from build123d import *

# Parameters (mm, degrees)
F0_R     = 2.3495
F0_R_2   = 3.96875
F0_W     = 15.748
F0_H     = 17.272
F0_W_2   = 48.387
F0_H_2   = 25.781
F0_R_3   = 7.14375
F1_DEPTH = 6.35


with BuildPart() as f1:
    # F0 (on Top) → F1 (new body)
    with BuildSketch(Plane.XY):
        with BuildLine():
            ThreePointArc((61.595, 55.245), (59.735128, 59.735128), (55.245, 61.595))
            Line((55.245, 61.595), (-55.245, 61.595))
            ThreePointArc((-55.245, 61.595), (-59.735128, 59.735128), (-61.595, 55.245))
            Line((-61.595, 55.245), (-61.595, -55.245))
            ThreePointArc((-61.595, -55.245), (-59.735128, -59.735128), (-55.245, -61.595))
            Line((-55.245, -61.595), (55.245, -61.595))
            ThreePointArc((55.245, -61.595), (59.735128, -59.735128), (61.595, -55.245))
            Line((61.595, -55.245), (61.595, 55.245))
        make_face()
        with Locations((-45.212, -41.402)):
            Circle(F0_R, mode=Mode.SUBTRACT)
        with Locations((-29.845, -23.495)):
            Circle(F0_R_2, mode=Mode.SUBTRACT)
        with Locations((10.795, -33.02)):
            Circle(F0_R_2, mode=Mode.SUBTRACT)
        with Locations((45.212, -41.402)):
            Circle(F0_R, mode=Mode.SUBTRACT)
        with Locations((29.845, -23.495)):
            Circle(F0_R_2, mode=Mode.SUBTRACT)
        with Locations((10.795, -13.97)):
            Circle(F0_R_2, mode=Mode.SUBTRACT)
        with Locations((-29.845, 20.32)):
            Rectangle(F0_W, F0_H, mode=Mode.SUBTRACT)
        with Locations((-45.212, 41.402)):
            Circle(F0_R, mode=Mode.SUBTRACT)
        with Locations((10.795, 20.32)):
            Rectangle(F0_W_2, F0_H_2, mode=Mode.SUBTRACT)
        with Locations((0, 50.224401)):
            Circle(F0_R_3, mode=Mode.SUBTRACT)
        with Locations((45.212, 41.402)):
            Circle(F0_R, mode=Mode.SUBTRACT)
    extrude(amount=F1_DEPTH)


solid = f1.part
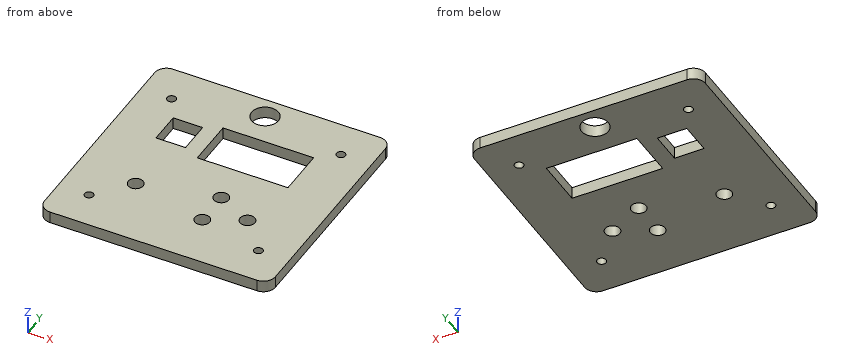
Could you check a few things on this model? Use its own coordinates, in mm. Give positions to 0.01 mm unless a question says otherwise; leave off trailing zeros. Order: outer loops, then holes, each group sorted by start corner. A loop starts at its lowest first (then second) coordinate and runs counter-clockwise, first axis right, second up.
1. Suppose I cut it at C-C (y = -13.97). Write out the boundary of the cut face in (x, z) (3 decimals), plus the area to 3 significant figures.
Answers below:
outline: (-61.595, 0) - (6.826, 0) - (6.826, 6.35) - (-61.595, 6.35) - close; (14.764, 0) - (61.595, 0) - (61.595, 6.35) - (14.764, 6.35) - close
area: 732 mm2
2. Suppose I cut it at A-A (y = 20). State how many separate pieces and enclosed holes the cut face has, plus the area to 3 significant figures.
Answers below:
separate pieces: 3
enclosed holes: 0
area: 375 mm2
3. For pin 1 (5.5 mm diameter, centred on x = 45.212, y = 41.402, fed in from +Z), with a flat end and sliding along its axis, tell me the tip position at first contact or that it passes through.
Answers below:
pin 1: stops at z = 6.35
4. I need wall thicknesses on L1, parallel to Y at x = 0, z = 2 (1 decimal); L2, parallel to Y at x = 30, z = 2.5 (1 decimal); L3, parallel to X at y = 18, z = 0.5 (1 decimal). Which ranges of each line are inside material? Lowest first, please.
Answers below:
L1: y = -61.6 to 7.4, 33.2 to 43.1, 57.4 to 61.6
L2: y = -61.6 to -27.5, -19.5 to 7.4, 33.2 to 61.6
L3: x = -61.6 to -37.7, -22 to -13.4, 35 to 61.6
